Here's how the part is built. I have some questions about the finished solid (model axes, mm). A direction names the side the tool comes from. Give positions to 0.01 mm unless a question says otherwise; leave off trailing zeros. Order: outer loops, then holes, each group sorted by start corner. A loop starts at its lowest first (then second) coordinate and runs counter-clockwise, first axis right, second up.
from build123d import *

# Parameters (mm, degrees)
F1_DEPTH = 10


with BuildPart() as f1:
    # F0 (on Front) → F1 (new body)
    with BuildSketch(Plane.XZ):
        Polygon((-17.288136, 10), (-17.288136, 0), (62.711864, 0), (62.711864, 10), (42.711864, 10), (34.830804, 10), (11.184005, 10), (2.711864, 10), align=None)
        Polygon((2.711864, 18.67337), (2.711864, 10), (11.184005, 10), (11.184005, 28.67337), (2.711864, 28.67337), align=None)
        Polygon((34.830804, 10), (42.711864, 10), (42.711864, 18.67337), (42.711864, 28.67337), (34.830804, 28.67337), align=None)
        Polygon((-7.288136, 18.67337), (2.711864, 18.67337), (2.711864, 28.67337), (2.711864, 98.67337), (-7.288136, 98.67337), align=None)
        Polygon((42.711864, 28.67337), (42.711864, 18.67337), (52.711864, 18.67337), (52.711864, 98.67337), (42.711864, 98.67337), align=None)
    extrude(amount=F1_DEPTH)


solid = f1.part
Q1. I need wall thicknesses on L1, parallel to X at y = -9.5, z = 30; L2, parallel to Z at x = -1.5, y = -9; L3, parallel to X at y = -8, z = 17.5. Which ranges of each line are inside material? Lowest first, please.
Filled sheet:
L1: x = -7.29 to 2.71, 42.71 to 52.71
L2: z = 0 to 10, 18.67 to 98.67
L3: x = 2.71 to 11.18, 34.83 to 42.71
Q2. If we section it at A-A on z = 13.5: List the corners of the cut face in (x, y) for me.
Filled sheet:
outline: (2.71, -10) - (11.18, -10) - (11.18, 0) - (2.71, 0) - close; (34.83, -10) - (42.71, -10) - (42.71, 0) - (34.83, 0) - close
Q3. If we section it at D-D on x = 21: List the corners of the cut face in (y, z) for me, plus the area to 3 significant figures.
Filled sheet:
outline: (-10, 0) - (0, 0) - (0, 10) - (-10, 10) - close
area: 100 mm2
Q4. If we section it at B-B on x = 51: List the corners of the cut face in (y, z) for me.
Filled sheet:
outline: (-10, 0) - (0, 0) - (0, 10) - (-10, 10) - close; (-10, 18.67) - (0, 18.67) - (0, 98.67) - (-10, 98.67) - close
Q5. I'm going to push flat-ended pins straight in: P1, Ø5, axis at y = -6.5, z = 17.5, coming from the -X side; P2, Ø4.5, axis at y = -4.5, z = 14, coming from the -X side; P3, Ø3, axis at y = -5, z = 60.5, coming from the +X side; P4, Ø1, axis at x = -8, z = 83, coming from the +Y side. Where does each tip first touch, or does it pass through?
Filled sheet:
P1: stops at x = -7.29
P2: stops at x = 2.71
P3: stops at x = 52.71
P4: passes through
Q6. If we section it at C-C on y = -3.25: List the corners of the cut face in (x, z) for me.
Filled sheet:
outline: (-17.29, 0) - (62.71, 0) - (62.71, 10) - (42.71, 10) - (42.71, 18.67) - (52.71, 18.67) - (52.71, 98.67) - (42.71, 98.67) - (42.71, 28.67) - (34.83, 28.67) - (34.83, 10) - (11.18, 10) - (11.18, 28.67) - (2.71, 28.67) - (2.71, 98.67) - (-7.29, 98.67) - (-7.29, 18.67) - (2.71, 18.67) - (2.71, 10) - (-17.29, 10) - close
Q7. Thinking about a two-plate mould opening in X: for faces 1 (the face through (48, -5, 98.673)), 2 (the face through (42.712, -5, 14)), 3 (the face through (11.184, -5, 19)), which applies, released by +X, released by -X, zero draft, split by the parting line, or undercut?
Filled sheet:
face 1: zero draft
face 2: released by +X
face 3: undercut
Q8. For faces 4 (the face through (52.712, -5, 58)), 5 (the face through (-7, -5, 10)), 6 (the face through (7, -5, 28.673)), which set-ups out of +Z, -Z, +X, -X, +Y, -Y let a thin tool reach every point of the face, with its end or its side?
Filled sheet:
face 4: +Z, +X, +Y, -Y
face 5: -X, +Y, -Y
face 6: +Z, +Y, -Y
